Could you check a few things on this model? Use its own coordinates, in mm. Face numbers are marked on the shaded views. Give positions to 0.01 mm unless a question says otherwise; leave off trailing zeros. Write each loop counter-clockwise with the first axis right and the second up, starting at its lowest first coordinate (ties: lowest second). Pieces come first, ordered by that corner, then holes. Notation, with made-up numbers: (47.5, 24.25) - (53.5, 24.25) arc R19 ccw to (53.5, 28.25) - close; hole circle Ø6 at (42.25, -13). An arc over 180 degrees is marked (long way). Answer as a JSON object with one key per item and string values. Group by question number.
```python
from build123d import *

# Parameters (mm, degrees)
ESQUISSE1_R             = 54.5
ESQUISSE1_R_2           = 47.5
BOSS_EXTRU_1_DEPTH      = 15
ESQUISSE2_W             = 1
ESQUISSE2_H             = 9.520304005
ENL_V_MAT_EXTRU_1_DEPTH = 6


with BuildPart() as part:
    # Esquisse1 → Boss.-Extru.1 (new body)
    with BuildSketch(Plane.XY):
        Circle(ESQUISSE1_R)
        Circle(ESQUISSE1_R_2, mode=Mode.SUBTRACT)
    extrude(amount=BOSS_EXTRU_1_DEPTH)

    # Esquisse2 → Enlèv. mat.-Extru.1 (cut)
    with BuildSketch(Plane(origin=(0, 0, 0), x_dir=(-1, 0, 0), z_dir=(0, 0, -1))):
        with BuildLine():
            Line((32.437456587, -43.795677985), (28.322761135, -38.132285556))
            ThreePointArc((28.322761135, -38.132285556), (27.919799484, -38.428307233), (27.513744141, -38.720070808))
            Line((27.513744141, -38.720070808), (31.628439593, -44.383463237))
            ThreePointArc((31.628439593, -44.383463237), (32.03429625, -44.091426193), (32.437456587, -43.795677985))
        make_face()
        with BuildLine():
            ThreePointArc((-45.327190172, 14.20196575), (-45.175184524, 14.678307233), (-45.018173177, 15.153022266))
            Line((-45.018173177, 15.153022266), (-51.675890273, 17.316245682))
            ThreePointArc((-51.675890273, 17.316245682), (-51.832580138, 16.841426193), (-51.984907267, 16.365189166))
            Line((-51.984907267, 16.365189166), (-45.327190172, 14.20196575))
        make_face()
        Polygon((-26.511777811, -37.340982466), (-32.107672102, -45.043070198), (-32.916689096, -44.455284946), (-27.320794805, -36.753197214), align=None)
        Polygon((43.3969576, 14.626257393), (52.451304761, 17.568193122), (52.760321755, 16.617136606), (43.705974594, 13.675200877), align=None)
        with Locations((0, 50.552873414)):
            Rectangle(ESQUISSE2_W, ESQUISSE2_H)
    extrude(amount=-ENL_V_MAT_EXTRU_1_DEPTH, mode=Mode.SUBTRACT)


solid = part.part
```
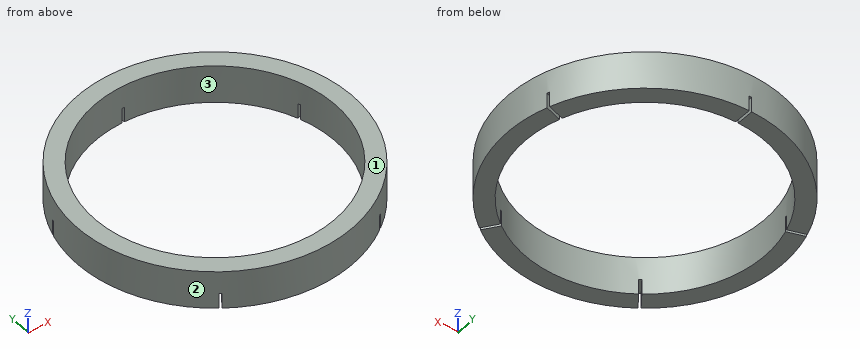
(1) I need wall thicknesses on L1, parallel to Y at x = 0, z = 10.25; L2, parallel to X at y = -40, z = 3.5. Which ranges of each line are inside material? Lowest first, please.
(2) If we mould it in two halves opening along Y, with no side actions, what happens to the marked faces 1, 2 and 3? For each: +Y half, -Y half, draft (parallel to the pull), parting line (faces both ways), or undercut.
(3) I want a section at A-A, the plane y = 0. Please give me the cut outline in (x, z), and give its area (3 significant figures).
(4) Will these pins go through, and if not, where does the flat tip stop? P1, Ø0.9, axis at x = -49.5, y = 16.5, coming from the -Z side; P2, Ø8, axis at x = -12, z = 2, coming from the -Y side; P3, Ø4, axis at y = 17, z = 3, coming from the -X side; P4, Ø1.8, axis at y = 51, z = 3.5, coming from the -X side.
(5) I want a section at C-C, the plane z = 12.75. Please give me the cut outline in (x, y), and give its area (3 significant figures).
(6) I want a section at B-B, the plane x = 34. Please give me the cut outline in (y, z), and give its area (3 significant figures).
Entries:
{
 "1": {"L1": "-54.5 to -47.5, 47.5 to 54.5", "L2": "-37.02 to -29.68, -28.44 to -25.62, 25.62 to 28.44, 29.68 to 37.02"},
 "2": {"face 1": "draft", "face 2": "parting line", "face 3": "undercut"},
 "3": {"outline": "(-54.5, 0) - (-47.5, 0) - (-47.5, 15) - (-54.5, 15) - close; (47.5, 0) - (54.5, 0) - (54.5, 15) - (47.5, 15) - close", "area": "210 mm^2"},
 "4": {"P1": "z = 0", "P2": "y = -53.91", "P3": "x = -52.4", "P4": "x = -21.45"},
 "5": {"outline": "circle Ø109 at (0, 0); hole circle Ø95 at (0, 0)", "area": "2,240 mm^2"},
 "6": {"outline": "(-42.59, 0) - (-33.17, 0) - (-33.17, 15) - (-42.59, 15) - close; (33.17, 0) - (42.59, 0) - (42.59, 15) - (33.17, 15) - close", "area": "283 mm^2"}
}
